from build123d import *

# Parameters (mm, degrees)
F0_R     = 30
F0_R_2   = 6
F1_DEPTH = 4
F2_DEPTH = 6
F3_R     = 1.5
F4_DEPTH = 12.5
F5_W     = 3
F5_H     = 4.6
F6_DEPTH = 9.4


with BuildPart() as f1:
    # F0 (on Top) → F1 (new body)
    with BuildSketch(Plane.XY):
        Circle(F0_R)
        Circle(F0_R_2, mode=Mode.SUBTRACT)
        Circle(F0_R_2)
    extrude(amount=-F1_DEPTH)

    # F0 (on Top) → F2 (join)
    with BuildSketch(Plane.XY):
        Circle(F0_R_2)
    extrude(amount=F2_DEPTH)

    # F3 (on Front) → F4 (cut, symmetric)
    with BuildSketch(Plane.XZ):
        with Locations((0, 3)):
            Circle(F3_R)
    extrude(amount=F4_DEPTH, both=True, mode=Mode.SUBTRACT)

    # F5 (on face) → F6 (cut)
    with BuildSketch(Plane.XY.offset(6)):
        Rectangle(F5_W, F5_H)
        with BuildLine():
            Line((-1.5, 2.3), (1.5, 2.3))
            ThreePointArc((1.5, 2.3), (0, 2.7540939565), (-1.5, 2.3))
        make_face()
        with BuildLine():
            ThreePointArc((-1.5, -2.3), (0, -2.7459060435), (1.5, -2.3))
            Line((1.5, -2.3), (-1.5, -2.3))
        make_face()
    extrude(amount=-F6_DEPTH, mode=Mode.SUBTRACT)

    # F7 (on Front) → F8 (revolve, cut)
    with BuildSketch(Plane.XZ):
        Polygon((-28.5857864376, -2), (-30, -0.5857864376), (-30, -3.4142135624), align=None)
    revolve(axis=Axis((0, 0, 0.2672639675), (0, 0, -1)), mode=Mode.SUBTRACT)


solid = f1.part
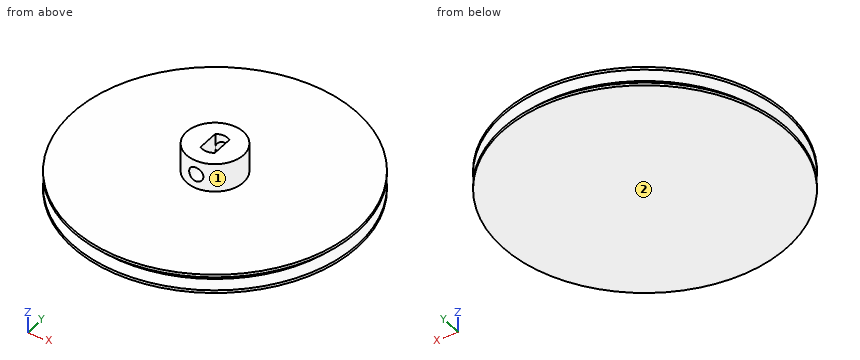
The model under review builds one solid part; all positions refer to its coordinate system, in mm. Face numbers are marked on the shaded views. A direction names the side the tool comes from. Give positions to 0.01 mm unless a question says otherwise; leave off trailing zeros. Order: outer loops, then holes, each group sorted by start corner. A loop starts at its lowest first (then second) coordinate and runs counter-clockwise, first axis right, second up. Notation, with made-up numbers: M -37.5,-30.5 L -25.5,-30.5 A11 ccw -25.5,-26.5 Z; hole C 80,34 d9. An arc over 180 degrees is marked long. Use one line per item in the form item = value. Start each with the question number.
Item 1: We need section B-B on z = 2.25. Give the boundary of the cut face in (x, y).
Item 2: We need section C-C on y = 0. Give the boundary of the cut face in (x, z), plus the area to 3 significant figures.
Item 3: We need section A-A on x = 0. Give the boundary of the cut face in (y, z).
Item 4: To check wall thickness, follow line 1 along Z through (x, y) = (0, 3); line 2 along Y through (x, z) = (0, -0.5); line 3 along Z through (x, y) = (-3.5, -5.5). State the ranges of each line that lie inside material, in increasing order. Write a range as from..to.
Item 5: For the marked faces 1 and 2, list the 3-axis set-ups (+Z, -Z, +X, -X, +Y, -Y) from which the entire face can be reached by the end or side of a thin tool; tool diameter is ignored.
Item 6: Insertion check: pin 1 Ø5 at (y, z) = (-21.5, 3) entering from -X; pin 2 Ø1.5 at (x, z) = (8.5, -2.5) entering from -Y; pin 3 Ø2.5 at (y, z) = (-0.5, 3) entering from -X; pin 4 Ø2 at (y, z) = (21.5, -1.5) entering from +X. Each pin has a flat end and moves straight along its axis. Give the tip position at first contact, or say it passes through.
Completed:
q1.outline = M -1.5,-2.3 L -1.5,2.3 A2.7 cw -1.3,2.42 L -1.3,5.86 A6 ccw -1.3,-5.86 L -1.3,-2.42 A2.75 cw Z; M 1.3,-5.86 A6 ccw 1.3,5.86 L 1.3,2.42 A2.7 cw 1.5,2.3 L 1.5,-2.3 A2.75 cw 1.3,-2.42 Z
q2.outline = M -30,-4 L 30,-4 L 30,-3.41 L 28.59,-2 L 30,-0.59 L 30,0 L 6,0 L 6,6 L 1.5,6 L 1.5,-3.4 L -1.5,-3.4 L -1.5,6 L -6,6 L -6,0 L -30,0 L -30,-0.59 L -28.59,-2 L -30,-3.41 Z
q2.area = 280 mm²
q3.outline = M -30,-4 L 30,-4 L 30,-3.41 L 28.59,-2 L 30,-0.59 L 30,0 L 6,0 L 6,1.5 L 2.75,1.5 L 2.75,-3.4 L -2.75,-3.4 L -2.75,1.5 L -6,1.5 L -6,0 L -30,0 L -30,-0.59 L -28.59,-2 L -30,-3.41 Z; M -6,4.5 L -2.75,4.5 L -2.75,6 L -6,6 Z; M 2.75,4.5 L 6,4.5 L 6,6 L 2.75,6 Z
q4.line_1 = -4..1.5, 4.5..6
q4.line_2 = -30..-2.75, 2.75..30
q4.line_3 = -4..0
q5.face_1 = +Z
q5.face_2 = -Z, +X, -X, +Y, -Y
q6.pin_1 = through
q6.pin_2 = -28.63
q6.pin_3 = -6
q6.pin_4 = 21.36
